Design review of the part built by this model. Coordinates are the model's own, in mm. A direction names the side the tool comes from. Give positions to 0.01 mm unless a question says otherwise; leave off trailing zeros. Loops run counter-clockwise (first coordinate to the right, second up) from the corner with the lowest first, then second, coordinate; pieces in that order, holes last. Notation, with made-up numbers: (13.25, 72.25) - (20.25, 72.25) arc R23 ccw to (20.25, 91.25) - close; hole circle Ø6 at (64, 13.25). An arc over 180 degrees is marked (long way). Write each question's results on one line, items separated by ' | '.
Autodesk Inventor part; units mm, degrees
ref_plane "YZ Plane" through (0, 0, 0) normal (1, 0, 0) x (0, 1, 0)
ref_plane "XZ Plane" through (0, 0, 0) normal (0, 1, 0) x (-1, 0, 0)
ref_plane "XY Plane" through (0, 0, 0) normal (0, 0, 1) x (1, 0, 0)
sketch "Sketch2" plane through (0, 0, 0) normal (0, 0, 1) x (1, 0, 0)
  line L0 (-12.7, -12.7) -> (12.7, -12.7)
  line L1 (12.7, -12.7) -> (12.7, 12.7)
  line L2 (12.7, 12.7) -> (-12.7, 12.7)
  line L3 (-12.7, 12.7) -> (-12.7, -12.7)
  line L4 (-12.7, -12.7) -> (12.7, 12.7) construction
  line L5 (12.7, -12.7) -> (-12.7, 12.7) construction
  line L6 (-9.525, -9.525) -> (9.525, -9.525)
  line L7 (9.525, -9.525) -> (9.525, 9.525)
  line L8 (9.525, 9.525) -> (-9.525, 9.525)
  line L9 (-9.525, 9.525) -> (-9.525, -9.525)
  line L10 (-9.525, -9.525) -> (9.525, 9.525) construction
  line L11 (9.525, -9.525) -> (-9.525, 9.525) construction
  point P0 (0, 0)
  dimension "d0" = 25.4
  dimension "d1" = 25.4
  dimension "d2" = 3.175
  dimension "d3" = 3.175
extrude "Extrusion1" add sketch "Sketch2" along normal mid plane 601.2155
sketch "Sketch3" plane through (12.7, -12.7, 300.6077) normal (1, 0, 0) x (0, 0, -1)
  line L0 (601.2155, 0) -> (0, 0)
  line L1 (0, 0) -> (43.9941, 25.4)
  line L2 (601.2155, 25.4) -> (0, 25.4)
  line L3 (43.9941, 25.4) -> (0, 25.4)
  line L4 (0, 0) -> (0, 25.4)
  line L5 (0, 3.175) -> (601.2155, 3.175)
  point P0 (300.6077, 12.7)
  dimension "d6" = 30
extrude "Extrusion2" cut sketch "Sketch3" against normal through all
sketch "Sketch5" plane through (12.7, -12.7, -300.6077) normal (1, 0, 0) x (0, 0, -1)
  line L0 (0, 0) -> (-25.4, 25.4)
  line L1 (-557.2214, 25.4) -> (0, 25.4)
  line L2 (0, 0) -> (-601.2155, 0)
  line L3 (-25.4, 25.4) -> (0, 25.4)
  line L4 (0, 0) -> (0, 25.4)
  line L5 (0, 25.4) -> (0, 0)
  point P0 (-300.6077, 12.7)
  dimension "d10" = 45
extrude "Extrusion3" cut sketch "Sketch5" against normal through all
properties part number "aluminumBallHandlerBase" material "Aluminum 6061-AHC"
Item 1: Tool access review of faces 4 (the face through (-9.525, 0, -5)), 5 (the face through (0, 12.7, -13)): name each direction out of +Z, -Z, +X, -X, +Y, -Y from which nothing blocks a thin tool from reaching the whole face with its end or side.
Output values:
face 4: +Z, -Z | face 5: +Z, -Z, +X, -X, +Y
Item 2: Clearance check with flat-ended pins moving along their axes: P1, Ø6, axis at x = 2, y = -7, coming from the -Z side; P2, Ø10, axis at x = 5, y = 7.5, coming from the -Z side; P3, Ø4, axis at x = 9.5, y = 4, coming from the -Z side; P4, Ø6, axis at x = -5, y = -3, coming from the +Z side. State where each tip first meets the part, or that it passes through.
Output values:
P1: stops at z = -297.91 | P2: stops at z = -282.53 | P3: stops at z = -285.91 | P4: passes through
Item 3: We need section B-B on z = 246. Give the boundary of the cut face in (x, y) (3 decimals).
Output values:
outline: (-12.7, -12.7) - (12.7, -12.7) - (12.7, 12.7) - (-12.7, 12.7) - close; hole (-9.525, -9.525) - (9.525, -9.525) - (9.525, 9.525) - (-9.525, 9.525) - close
Item 4: We need section C-C on y = -0.25. Give the boundary of the cut face in (x, z) (3 decimals).
Output values:
outline: (-12.7, -288.158) - (-9.525, -288.158) - (-9.525, 279.044) - (-12.7, 279.044) - close; (9.525, -288.158) - (12.7, -288.158) - (12.7, 279.044) - (9.525, 279.044) - close
Item 5: We need section A-A on x = 5.5. Give the boundary of the cut face in (y, z) (3 decimals).
Output values:
outline: (-12.7, -300.608) - (-9.525, -297.433) - (-9.525, 295.108) - (-12.7, 300.608) - close; (9.525, -278.383) - (12.7, -275.208) - (12.7, 256.614) - (9.525, 262.113) - close
Item 6: Wall thickness on probe 1 along X at (y, z) = (-4, -146) (3 decimals); probe 2 along Z at (x, y) = (-3, 9.75): over which ranges is each line inside the solid? List them lowest first.
Output values:
probe 1: x = -12.7 to -9.525, 9.525 to 12.7 | probe 2: z = -278.16 to 261.72
Item 7: Draft analysis for pull direction X (two halves, no side actions). For faces 1 (the face through (0, -12.7, -4)), 2 (the face through (9.525, 0, -5)), 3 (the face through (-12.7, 0, -4)), state which applies: +X half, -X half, draft (parallel to the pull), parting line (faces both ways), or undercut.
Output values:
face 1: draft | face 2: undercut | face 3: -X half
